The listing builds one solid part. Answer for the finished solid, in the listing's coordinates (mm). Face numbers are marked on the shaded views. A direction names the side the tool comes from. Coordinates: 2 decimals unless noted, no trailing zeros. Write each loop counter-clockwise with the first axis right and the second up, starting at its lowest first coordinate (ties: lowest second). Pieces come first, ordered by that corner, then holes.
from build123d import *

# Parameters (mm, degrees)
EXTRUDE_1_DEPTH     = 20
SKETCH_4_R          = 3
CUT_EXTRUDE_1_DEPTH = 10
SKETCH_5_R          = 2.5
CUT_EXTRUDE_2_DEPTH = 11


with BuildPart() as part:
    # 草圖1 → 填料-伸長1 (new body, symmetric)
    with BuildSketch(Plane.XY):
        Polygon((0, 0), (84, 0), (84, -10), (-16, -10), (-16, 57), (-13, 57), (-13, 60), (-3, 60), (-3, 57), (0, 57), align=None)
    extrude(amount=EXTRUDE_1_DEPTH, both=True)

    # 草圖4 → 除料-伸長1 (cut)
    with BuildSketch(Plane(origin=(0, 60, 0), x_dir=(1, 0, 0), z_dir=(0, 1, 0))):
        with Locations((-8, 10)):
            Circle(SKETCH_4_R)
        with Locations((-8, -10)):
            Circle(SKETCH_4_R)
    extrude(amount=-CUT_EXTRUDE_1_DEPTH, mode=Mode.SUBTRACT)

    # 草圖5 → 除料-伸長2 (cut, through all)
    with BuildSketch(Plane(origin=(0, 0, 0), x_dir=(1, 0, 0), z_dir=(0, 1, 0))):
        with Locations((40, -12.5)):
            Circle(SKETCH_5_R)
        with Locations((40, 12.5)):
            Circle(SKETCH_5_R)
        with Locations((75, 12.5)):
            Circle(SKETCH_5_R)
        with Locations((75, -12.5)):
            Circle(SKETCH_5_R)
        with BuildLine():
            Line((84, 7), (54, 7))
            ThreePointArc((54, 7), (47, 0), (54, -7))
            Line((54, -7), (84, -7))
            Line((84, -7), (84, 7))
        make_face()
    extrude(amount=-CUT_EXTRUDE_2_DEPTH, mode=Mode.SUBTRACT)


solid = part.part
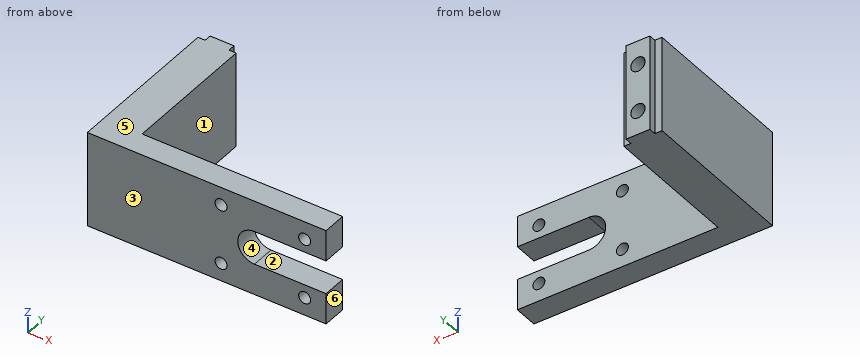
1. A tool of negligible diameter and unlimited length cuts with its end or side. For the marked faces 1, 2 and 3, from which of +Z, -Z, +X, -X, +Y, -Y can it reach the whole face along a straight path? Write none if from no direction.
Results found:
face 1: +Z, -Z, +X, +Y
face 2: +X, +Y, -Y
face 3: +Z, -Z, +X, -X, -Y
2. Section C-C on z = 0 is taken. Give the vertices of the cut face in (x, y).
Results found:
outline: (-16, -10) - (47, -10) - (47, 0) - (0, 0) - (0, 57) - (-3, 57) - (-3, 60) - (-13, 60) - (-13, 57) - (-16, 57) - close
3. Flat-ended cylindrical pins translate along their axes: P1, Ø8, axis at y = 4.5, z = -3, coming from the +X side; P2, Ø10, axis at x = 17.5, z = 0, coming from the +Y side; P3, Ø3, axis at x = 75, z = 12.5, coming from the +Y side; P4, Ø2.5, axis at y = 59, z = -8.5, coming from the +X side. Find the tip coordinate at first contact, or state that the pin passes through.
Results found:
P1: stops at x = 0
P2: stops at y = 0
P3: passes through
P4: stops at x = -3
4. Section A-A on x = 75 is taken. Give the vertices of the cut face in (y, z).
Results found:
outline: (-10, -20) - (0, -20) - (0, -15) - (-10, -15) - close; (-10, -10) - (0, -10) - (0, -7) - (-10, -7) - close; (-10, 7) - (0, 7) - (0, 10) - (-10, 10) - close; (-10, 15) - (0, 15) - (0, 20) - (-10, 20) - close
5. For a pull along Z with two mould halves and no side action, classify the marked faces 4, 5 and 6 as pulls with the +Z half, pulls with the -Z half, needs draft (parallel to the pull), parting line crosses it, or undercut.
Results found:
face 4: undercut
face 5: pulls with the +Z half
face 6: needs draft
6. Section D-D on y = 52 is taken. Give the vertices of the cut face in (x, z), then the cut area to 3 significant figures.
Results found:
outline: (-16, -20) - (0, -20) - (0, 20) - (-16, 20) - close; hole circle Ø6 at (-8, -10); hole circle Ø6 at (-8, 10)
area: 583 mm2
7. Section B-B on y = -4.5 is taken. Give the vertices of the cut face in (x, z).
Results found:
outline: (-16, -20) - (84, -20) - (84, -7) - (54, -7) arc R7 cw to (54, 7) - (84, 7) - (84, 20) - (-16, 20) - close; hole circle Ø5 at (40, -12.5); hole circle Ø5 at (40, 12.5); hole circle Ø5 at (75, -12.5); hole circle Ø5 at (75, 12.5)
8. Find the intervals of material crossed by L1, parallel to X at y = -7.75, z = -12.5; L2, parallel to Z at x = 40, y = -4; L3, parallel to Z at x = 75, y = -4, in increasing order.
Results found:
L1: x = -16 to 37.5, 42.5 to 72.5, 77.5 to 84
L2: z = -20 to -15, -10 to 10, 15 to 20
L3: z = -20 to -15, -10 to -7, 7 to 10, 15 to 20
